Part model, mm, in its own coordinate system. A direction names the side the tool comes from. Give positions to 0.01 mm unless a question says otherwise; leave off trailing zeros. Loops run counter-clockwise (first coordinate to the right, second up) from the corner with the lowest first, then second, coordinate; pieces in that order, holes last. Notation, with made-up numbers: M 52,-9 L 102,-9 A24 ccw 102,2 Z; hole C 48,53.25 d3. An arc over 180 degrees is marked long. Answer in a Markdown table with one row per item.
from build123d import *

# Parameters (mm, degrees)
F1_DEPTH  = 400
F2_T      = -20
F4_DEPTH  = 40
F5_W      = 40
F5_H      = 61.2435565298
F6_DEPTH  = 5
F7_W      = 5
F7_H      = 61.2435565298
F8_DEPTH  = 40
F9_W      = 20
F9_H      = 41.2435565298
F10_DEPTH = 20


with BuildPart() as f1:
    # F0 (on Front) → F1 (new body)
    with BuildSketch(Plane.XZ):
        Polygon((175.5110102277, 79.7711170535), (-124.4889897723, 79.7711170535), (-274.4889897723, -180.0365040818), (-124.4889897723, -439.8441252172), (175.5110102277, -439.8441252172), (325.5110102277, -180.0365040818), align=None)
    extrude(amount=F1_DEPTH)

    # F2
    f2_openings = [f1.faces().sort_by_distance(p)[0] for p in [
        (25.51101, -400, -180.036504),
    ]]
    offset(amount=F2_T, openings=f2_openings)

    # F3 (on face) → F4 (join)
    with BuildSketch(Plane.XZ.offset(400)):
        Polygon((175.5110102277, -439.8441252172), (325.5110102277, -180.0365040818), (175.5110102277, 79.7711170535), (-124.4889897723, 79.7711170535), (-274.4889897723, -180.0365040818), (-124.4889897723, -439.8441252172), align=None)
        Polygon((-216.3949790047, -240.6582823468), (-251.3949790047, -180.0365040818), (-216.3949790047, -119.4147258169), (-112.9419843885, 59.7711170535), (163.9640048439, 59.7711170535), (267.4169994601, -119.4147258169), (302.4169994601, -180.0365040818), (267.4169994601, -240.6582823468), (163.9640048439, -419.8441252172), (-112.9419843885, -419.8441252172), align=None, mode=Mode.SUBTRACT)
        Polygon((-216.3949790047, -119.4147258169), (-251.3949790047, -180.0365040818), (-216.3949790047, -240.6582823468), align=None)
        Polygon((302.4169994601, -180.0365040818), (267.4169994601, -119.4147258169), (267.4169994601, -240.6582823468), align=None)
    extrude(amount=-F4_DEPTH)

    # F5 (on face) → F6 (join)
    with BuildSketch(Plane.YZ.offset(-216.3949790047)):
        with Locations((-380, -180.0365040818)):
            Rectangle(F5_W, F5_H)
    extrude(amount=F6_DEPTH)

    # F7 (on face) → F8 (join)
    with BuildSketch(Plane.XZ.offset(400)):
        with Locations((-213.8949790047, -180.0365040818)):
            Rectangle(F7_W, F7_H)
    extrude(amount=F8_DEPTH)

    # F9 (on face) → F10 (cut)
    with BuildSketch(Plane(origin=(267.4169994601, 0, 0), x_dir=(0, -1, 0), z_dir=(-1, 0, 0))):
        with Locations((380.0858259201, -180.0365040818)):
            Rectangle(F9_W, F9_H)
    extrude(amount=-F10_DEPTH, mode=Mode.SUBTRACT)


solid = f1.part
(1) Saw through at C-C (z = -296.5). Write the cut outline in (x, y), plus the area to 3 significant figures.
Recorded:
| item | result |
|---|---|
| outline | M -207.25,-400 L -184.15,-400 L -184.15,-20 L 235.18,-20 L 235.18,-400 L 258.27,-400 L 258.27,0 L -207.25,0 Z |
| area | 26,900 mm^2 |
(2) Pin check, flat tips, straight feed: pin 1 Ø20 at (y, z) = (-424, -174.5) entering from -X (3 decimals); pin 2 Ø2 at (x, z) = (-171, -46.5) entering from -Y; pin 3 Ø22 at (x, y) = (274.5, -377) entering from +Z; pin 4 Ø1 at (x, z) = (80, -363) entering from +Y. Stop position of each tip, or through.
Recorded:
| item | result |
|---|---|
| pin 1 | stops at x = -216.395 |
| pin 2 | stops at y = -20 |
| pin 3 | stops at z = -72.63 |
| pin 4 | stops at y = 0 |
(3) Saw through at A-A (y = -201.5). Write the cut outline in (x, z), plus the area to 3 significant figures.
Recorded:
| item | result |
|---|---|
| outline | M -274.49,-180.04 L -124.49,-439.84 L 175.51,-439.84 L 325.51,-180.04 L 175.51,79.77 L -124.49,79.77 Z; hole M -251.39,-180.04 L -112.94,-419.84 L 163.96,-419.84 L 302.42,-180.04 L 163.96,59.77 L -112.94,59.77 Z |
| area | 34,600 mm^2 |
(4) Which spindle directions (+Z, -Z, +X, -X, +Y, -Y) get a long thin tool onto all of the face, cutting with end or side? Do faces 4 (the face through (24, -207, -419.844)), 5 (the face through (-216.395, -420, -180)), 6 (the face through (-183.14, -207.34, -298.26)). Say none if no direction does.
Recorded:
| item | result |
|---|---|
| face 4 | -Y |
| face 5 | +Z, -Z, -X, -Y |
| face 6 | none |
(5) Saw through at B-B (x = 118). Write the cut outline in (y, z), plus the area to 3 significant figures.
Recorded:
| item | result |
|---|---|
| outline | M -400,-439.84 L 0,-439.84 L 0,79.77 L -400,79.77 L -400,59.77 L -20,59.77 L -20,-419.84 L -400,-419.84 Z |
| area | 25,600 mm^2 |
(6) Pull direction Y, two halves, no side cores. Call faces 1 (the face through (269, -400, -179)), 2 (the face through (234.16, -207.34, -61.81)), 3 (the face through (-211.395, -399, -180)): +Y half, -Y half, draft (parallel to the pull), parting line (faces both ways), or undercut.
Recorded:
| item | result |
|---|---|
| face 1 | -Y half |
| face 2 | undercut |
| face 3 | draft |
(7) Drill centre lines: line 1 along Z through (x, y) = (98.5, -302.5); line 2 along Y through (x, z) = (-37, -306); line 3 along Y through (x, z) = (275.5, -241). Where is each one in solid material? Low to high.
Recorded:
| item | result |
|---|---|
| line 1 | z = -439.84 to -419.84, 59.77 to 79.77 |
| line 2 | y = -20 to 0 |
| line 3 | y = -400 to 0 |
